```python
from build123d import *

# Parameters (mm, degrees)
F0_W     = 1320.8
F0_H     = 304.8
F1_DEPTH = 19.05
F2_SIZE  = 19.04999
F3_W     = 1320.8
F3_H     = 19.05
F4_DEPTH = 9.525


# Not quite as in the source:
# - a fillet or chamfer is up to 0.001 mm smaller than in the source, because OpenCascade refuses the exact size


with BuildPart() as f1:
    # F0 (on Top) → F1 (new body)
    with BuildSketch(Plane.XY):
        with Locations((47.3523183346, -92.4993205261)):
            Rectangle(F0_W, F0_H)
    extrude(amount=F1_DEPTH)

    # F2 (size 19.05 in the source; OpenCascade refuses exactly that, so slightly less here)
    f2_edges = [f1.edges().sort_by_distance(p)[0] for p in [
        (707.752318, -92.499321, 19.05),
        (-613.047682, -92.499321, 19.05),
    ]]
    chamfer(f2_edges, length=F2_SIZE)

    # F3 (on face) → F4 (cut)
    with BuildSketch(Plane(origin=(0, 0, 0), x_dir=(1, 0, 0), z_dir=(0, 0, -1))):
        with Locations((47.3523183346, 209.9743205261)):
            Rectangle(F3_W, F3_H)
        with Locations((47.3523183346, -24.9756794739)):
            Rectangle(F3_W, F3_H)
    extrude(amount=-F4_DEPTH, mode=Mode.SUBTRACT)


solid = f1.part
```
Build history of the part. All positions in model axes, mm. Give positions to 0.01 mm unless a question says otherwise; leave off trailing zeros. Loops run counter-clockwise (first coordinate to the right, second up) from the corner with the lowest first, then second, coordinate; pieces in that order, holes last. Notation, with made-up numbers: (44, -18) - (97, -18) arc R33 cw to (97, 12) - close; hole circle Ø3 at (85.5, 76.5). An arc over 180 degrees is marked (long way). Use a Markdown table: item, result.
(1) Band-saw the part on A-A (z = 4.75). Give the cut face in (x, y), and give its area (3 significant figures).
Taken from the geometry:
| item | result |
|---|---|
| outline | (-608.3, -244.9) - (703, -244.9) - (703, -219.5) - (-608.3, -219.5) - close; (-608.3, -200.45) - (703, -200.45) - (703, 15.45) - (-608.3, 15.45) - close; (-608.3, 34.5) - (703, 34.5) - (703, 59.9) - (-608.3, 59.9) - close |
| area | 350,000 mm2 |
(2) Band-saw the part on B-B (x = -401.5). Give the cut face in (y, z) (3 decimals), and give its area (3 significant figures).
Taken from the geometry:
| item | result |
|---|---|
| outline | (-244.899, 0) - (-219.499, 0) - (-219.499, 9.525) - (-200.449, 9.525) - (-200.449, 0) - (15.451, 0) - (15.451, 9.525) - (34.501, 9.525) - (34.501, 0) - (59.901, 0) - (59.901, 19.05) - (-244.899, 19.05) - close |
| area | 5,440 mm2 |
(3) Wall check: line 1 along Y through (x, z) = (43, 8); line 2 along Z through (x, y) = (-443, 31.5) (3 decimals); line 3 along X through (y, z) = (-182, 9.5). Give the ranges that are in metal, low to high.
Taken from the geometry:
| item | result |
|---|---|
| line 1 | -244.9 to -219.5, -200.45 to 15.45, 34.5 to 59.9 |
| line 2 | 9.525 to 19.05 |
| line 3 | -603.55 to 698.25 |
(4) Drop flat-ended pins along their axis: pin 1 Ø5.5 at (x, y) = (212, -211.5) entering from -Z (3 decimals); pin 2 Ø6 at (y, z) = (11.5, 5.5) entering from +X; pin 3 Ø3 at (y, z) = (-49.5, 15) entering from -X. Give the stop position or say it passes through.
Taken from the geometry:
| item | result |
|---|---|
| pin 1 | z = 9.525 |
| pin 2 | x = 705.25 |
| pin 3 | x = -599.55 |
